Here's how the part is built. I have some questions about the finished solid (model axes, mm). Give positions to 0.01 mm unless a question says otherwise; leave off trailing zeros. Loops run counter-clockwise (first coordinate to the right, second up) from the corner with the lowest first, then second, coordinate; pieces in that order, holes last.
Q1. If we section it at D-D (y = 16.25): Please give me the cut outline in (x, z).
Q2. If we section it at A-A (z = 1.1): Give the number of separate pieces and of enclosed holes in the cut face, plus the area to 3 significant figures.
Q3. I need wall thicknesses on line 1 (Y direction, x = 9, z = 1.65); line 2 (X direction, y = 25, z = 0.65); line 3 (Y direction, x = 0, z = 2.15). Which ranges of each line are inside material? Lowest first, please.
Q4. If we section it at C-C (x = -9): Please give me the cut outline in (y, z).
Q5. If we section it at B-B (y = -7.75): Please give me the cut outline in (x, z).
Q6. Will this pin go through, and if not, where does the flat tip stop? P1, Ø4, axis at x = 9, y = -7.75, coming from the +Z side.
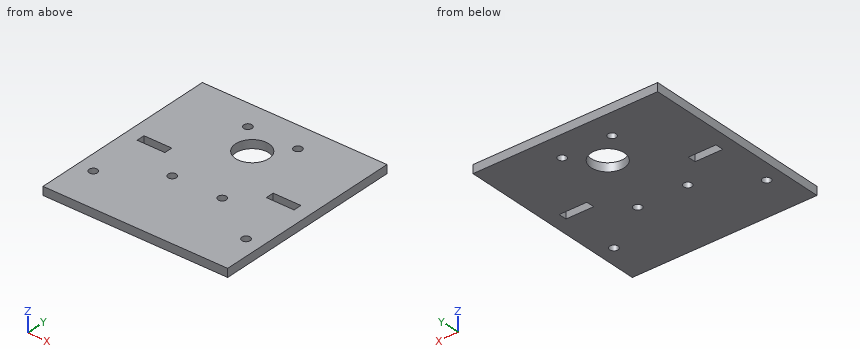
from build123d import *

# Parameters (mm, degrees)
SKETCH1_W           = 66.5
SKETCH1_H           = 69.5
BOSS_EXTRUDE1_DEPTH = 3
CUT_EXTRUDE1_REACH  = 50.188
SKETCH3_R           = 6
SKETCH3_R_2         = 1.5
CUT_EXTRUDE2_REACH  = 50.188
SKETCH4_R           = 1.5
CUT_EXTRUDE3_REACH  = 50.188
SKETCH5_W           = 10
SKETCH5_H           = 3


with BuildPart() as part:
    # Sketch1 → Boss-Extrude1 (new body)
    with BuildSketch(Plane.XY):
        Rectangle(SKETCH1_W, SKETCH1_H)
    extrude(amount=BOSS_EXTRUDE1_DEPTH)

    # Sketch3 → Cut-Extrude1 (cut, up to next)
    with BuildSketch(Plane.XY.offset(3), mode=Mode.PRIVATE) as cut_extrude1_sk1:
        with Locations((0, 16.25)):
            Circle(SKETCH3_R)
    cut_extrude1_tool1 = extrude(cut_extrude1_sk1.sketch, amount=-CUT_EXTRUDE1_REACH, mode=Mode.PRIVATE) & part.part
    # Sketch3 → Cut-Extrude1 (cut, up to next)
    with BuildSketch(Plane.XY.offset(3), mode=Mode.PRIVATE) as cut_extrude1_sk2:
        with Locations((9, 25.25)):
            Circle(SKETCH3_R_2)
    cut_extrude1_tool2 = extrude(cut_extrude1_sk2.sketch, amount=-CUT_EXTRUDE1_REACH, mode=Mode.PRIVATE) & part.part
    # Sketch3 → Cut-Extrude1 (cut, up to next)
    with BuildSketch(Plane.XY.offset(3), mode=Mode.PRIVATE) as cut_extrude1_sk3:
        with Locations((-9, 25.25)):
            Circle(SKETCH3_R_2)
    cut_extrude1_tool3 = extrude(cut_extrude1_sk3.sketch, amount=-CUT_EXTRUDE1_REACH, mode=Mode.PRIVATE) & part.part
    # Sketch3 → Cut-Extrude1 (cut, up to next)
    with BuildSketch(Plane.XY.offset(3), mode=Mode.PRIVATE) as cut_extrude1_sk4:
        with Locations((9, -7.75)):
            Circle(SKETCH3_R_2)
    cut_extrude1_tool4 = extrude(cut_extrude1_sk4.sketch, amount=-CUT_EXTRUDE1_REACH, mode=Mode.PRIVATE) & part.part
    # Sketch3 → Cut-Extrude1 (cut, up to next)
    with BuildSketch(Plane.XY.offset(3), mode=Mode.PRIVATE) as cut_extrude1_sk5:
        with Locations((-9, -7.75)):
            Circle(SKETCH3_R_2)
    cut_extrude1_tool5 = extrude(cut_extrude1_sk5.sketch, amount=-CUT_EXTRUDE1_REACH, mode=Mode.PRIVATE) & part.part
    add(cut_extrude1_tool1.solids().sort_by_distance((0, 16.25, 3))[0], mode=Mode.SUBTRACT)
    add(cut_extrude1_tool2.solids().sort_by_distance((9, 25.25, 3))[0], mode=Mode.SUBTRACT)
    add(cut_extrude1_tool3.solids().sort_by_distance((-9, 25.25, 3))[0], mode=Mode.SUBTRACT)
    add(cut_extrude1_tool4.solids().sort_by_distance((9, -7.75, 3))[0], mode=Mode.SUBTRACT)
    add(cut_extrude1_tool5.solids().sort_by_distance((-9, -7.75, 3))[0], mode=Mode.SUBTRACT)

    # Sketch4 → Cut-Extrude2 (cut, up to next)
    with BuildSketch(Plane.XY.offset(3), mode=Mode.PRIVATE) as cut_extrude2_sk1:
        with Locations((27.5, -19.75)):
            Circle(SKETCH4_R)
    cut_extrude2_tool1 = extrude(cut_extrude2_sk1.sketch, amount=-CUT_EXTRUDE2_REACH, mode=Mode.PRIVATE) & part.part
    cut_extrude2 = cut_extrude2_tool1.solids().sort_by_distance((27.5, -19.75, 3))[0]
    add(cut_extrude2, mode=Mode.SUBTRACT)

    # Mirror1: Cut-Extrude2 across plane
    add(cut_extrude2.mirror(Plane(origin=(0, 0, 0), x_dir=(0, 0, 1), z_dir=(1, 0, 0))), mode=Mode.SUBTRACT)

    # Sketch5 → Cut-Extrude3 (cut, up to next)
    with BuildSketch(Plane.XY.offset(3), mode=Mode.PRIVATE) as cut_extrude3_sk1:
        with Locations((23.25, 1.75)):
            Rectangle(SKETCH5_W, SKETCH5_H)
    cut_extrude3_tool1 = extrude(cut_extrude3_sk1.sketch, amount=-CUT_EXTRUDE3_REACH, mode=Mode.PRIVATE) & part.part
    cut_extrude3 = cut_extrude3_tool1.solids().sort_by_distance((23.25, 1.75, 3))[0]
    add(cut_extrude3, mode=Mode.SUBTRACT)

    # Mirror2: Cut-Extrude3 across plane
    add(cut_extrude3.mirror(Plane(origin=(0, 0, 0), x_dir=(0, 0, 1), z_dir=(1, 0, 0))), mode=Mode.SUBTRACT)


solid = part.part
Check sheet entries:
1. outline: (-33.25, 0) - (-6, 0) - (-6, 3) - (-33.25, 3) - close; (6, 0) - (33.25, 0) - (33.25, 3) - (6, 3) - close
2. separate pieces: 1
2. enclosed holes: 9
2. area: 4,410 mm2
3. line 1: y = -34.75 to -9.25, -6.25 to 23.75, 26.75 to 34.75
3. line 2: x = -33.25 to -10.48, -7.52 to 7.52, 10.48 to 33.25
3. line 3: y = -34.75 to 10.25, 22.25 to 34.75
4. outline: (-34.75, 0) - (-9.25, 0) - (-9.25, 3) - (-34.75, 3) - close; (-6.25, 0) - (23.75, 0) - (23.75, 3) - (-6.25, 3) - close; (26.75, 0) - (34.75, 0) - (34.75, 3) - (26.75, 3) - close
5. outline: (-33.25, 0) - (-10.5, 0) - (-10.5, 3) - (-33.25, 3) - close; (-7.5, 0) - (7.5, 0) - (7.5, 3) - (-7.5, 3) - close; (10.5, 0) - (33.25, 0) - (33.25, 3) - (10.5, 3) - close
6. P1: stops at z = 3
